```python
from build123d import *

# Parameters (mm, degrees)
SKETCH_R        = 8
SKETCH_R_2      = 6.5
PAD_DEPTH       = 40
SKETCH001_R     = 12
SKETCH001_R_2   = 6.5
PAD001_DEPTH    = 2
CHAMFER_SIZE    = 0.5
CHAMFER001_SIZE = 0.5


with BuildPart() as part:
    # Sketch → Pad (new body)
    with BuildSketch(Plane.XY):
        Circle(SKETCH_R)
        Circle(SKETCH_R_2, mode=Mode.SUBTRACT)
    extrude(amount=PAD_DEPTH)

    # Sketch001 → Pad001 (join)
    with BuildSketch(Plane.XY):
        Circle(SKETCH001_R)
        Circle(SKETCH001_R_2, mode=Mode.SUBTRACT)
    extrude(amount=PAD001_DEPTH)

    # Chamfer
    chamfer_edges = [part.edges().sort_by_distance(p)[0] for p in [
        (-8, 0, 40),
    ]]
    chamfer(chamfer_edges, length=CHAMFER_SIZE)

    # Chamfer001
    chamfer001_edges = [part.edges().sort_by_distance(p)[0] for p in [
        (-6.5, 0, 0),
    ]]
    chamfer(chamfer001_edges, length=CHAMFER001_SIZE)


solid = part.part
```
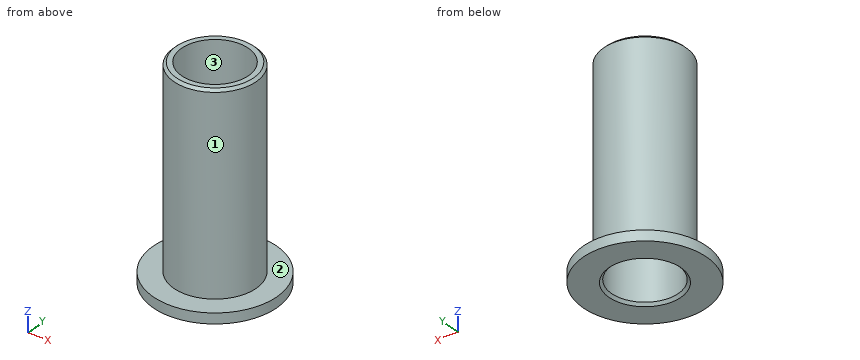
The listing builds one solid part. Answer for the finished solid, in the listing's coordinates (mm). Face numbers are marked on the shaded views. Give positions to 0.01 mm unless a question says otherwise; leave off trailing zeros. Loops run counter-clockwise (first coordinate to the right, second up) from the corner with the lowest first, then second, coordinate; pieces in that order, holes last. Notation, with made-up numbers: M 60,10.25 L 103,10.25 A13 cw 103,27.25 Z; hole C -15.75,87.25 d6. An arc over 180 degrees is marked long. One line per item, written item: value.
Q1. Find the intervals of material crossed by line 1 (Y direction, x = 0, z = 32.5); line 2 (Z direction, x = 8.5, y = 8); line 3 (X direction, y = -0.5, z = 32), in increasing order. Write a range as from..to.
Working result:
line 1: y = -8..-6.5, 6.5..8
line 2: z = 0..2
line 3: x = -7.98..-6.48, 6.48..7.98
Q2. Determine the mould class of the marked faces 1, 2 and 3 for opening direction Y: +Y half, -Y half, draft (parallel to the pull), parting line (faces both ways), or undercut.
Working result:
face 1: parting line
face 2: draft
face 3: undercut
Q3. Flat-ended cylindrical pins translate along their axes: P1, Ø4, axis at y = 2.5, z = 16.5, coming from the +X side; P2, Ø1.5, axis at x = 6, z = 15.5, coming from the -Y side; P3, Ø2, axis at y = -7.5, z = 17.5, coming from the -X side. Find the tip coordinate at first contact, or state that the pin passes through.
Working result:
P1: stops at x = 7.98
P2: stops at y = -6.04
P3: stops at x = -4.66
Q4. A cutting plane is placed at C-C on y = -10.25. Determine the outline of the cut face in (x, z).
Working result:
outline: M -6.24,0 L 6.24,0 L 6.24,2 L -6.24,2 Z
Q5. A cutting plane is placed at A-A on x = 0. Determine the outline of the cut face in (y, z).
Working result:
outline: M -12,0 L -7,0 L -6.5,0.5 L -6.5,40 L -7.5,40 L -8,39.5 L -8,2 L -12,2 Z; M 6.5,0.5 L 7,0 L 12,0 L 12,2 L 8,2 L 8,39.5 L 7.5,40 L 6.5,40 Z
Q6. A cutting plane is placed at B-B on z = 16.5. Determine the outline of the cut face in (x, y).
Working result:
outline: C 0,0 d16; hole C 0,0 d13
